Part model, mm, in its own coordinate system. A direction names the side the tool comes from. Coordinates: 2 decimals unless noted, no trailing zeros. Use a Markdown table: item, result. Add a question column.
1. Pull direction Y, two halves, no side cores. Call faces 3 (the flat face through (-5, 8, 0)), 4 (the flat face through (-6.4, 9.2, 0)), 5 (the cylindrical face through (-1.438, 10.955, -6.261)): pulls with the +Y half, pulls with the -Y half, needs draft (parallel to the pull), parting line crosses it, or undercut.
2. Drop flat-ended pins along their axis: pin 1 (10 mm diameter, centred on y = -9, z = 2, fed in from +X); pin 2 (6 mm diameter, centred on x = -5, z = 7, fed in from -Y); pin 3 (3 mm diameter, centred on y = -8, z = 37, fed in from +X). Give the stop position or say it passes through.
3. 3-axis set-ups, long thin cutter, end or side, ignore diameter. For faces 1 (the cylindrical face through (-1.88, -8.48, -6.26)), 2 (the flat face through (-7, -6, -12.7)): which of +Z, -Z, +X, -X, +Y, -Y reach the whole face in a straight line?
4. Wall check: probe 1 along Y at (x, z) = (0, -6.25); probe 2 along Y at (x, z) = (3.75, -2.5); probe 3 along X at (y, z) = (-8.5, 5). Give the ranges that are in metal, low to high. Write a range as [from, to].
from build123d import *

# Parameters (mm, degrees)
F2_R     = 11.049
F2_R_2   = 8.6868
F3_DEPTH = 12.7
F7_DEPTH = 3.302


# Not quite as in the source:
# - the program builds the solid bodies; features that only make, move or delete a surface that nothing else refers to are left out


with BuildPart() as f1:
    # F0 (on Front) → F1 (revolve)
    with BuildSketch(Plane.XZ):
        with BuildLine():
            Line((0, 59.2769769434), (0, 66.04))
            ThreePointArc((0, 66.04), (-9.3545638677, 33.6071762807), (-12.5095, 0))
            Line((-12.5095, 0), (-10.1473, 0))
            ThreePointArc((-10.1473, 0), (-7.5921575539, 30.0696179426), (0, 59.2769769434))
        make_face()
    revolve(axis=Axis((0, 0, 62.6584884717), (0, 0, 1)))

    # F2 (on Top) → F3 (join)
    with BuildSketch(Plane.XY):
        Circle(F2_R)
        Circle(F2_R_2, mode=Mode.SUBTRACT)
    extrude(amount=-F3_DEPTH)

    # F6 (on Front) → F7 (cut, symmetric)
    with BuildSketch(Plane.XZ):
        with BuildLine():
            ThreePointArc((6.9723, 0), (5.2204583943, 24.7022854782), (0, 48.9101079951))
            ThreePointArc((0, 48.9101079951), (-5.2204583943, 24.7022854782), (-6.9723, 0))
            Line((-6.9723, 0), (0, 0))
            Line((0, 0), (6.9723, 0))
        make_face()
    extrude(amount=F7_DEPTH, both=True, mode=Mode.SUBTRACT)


solid = f1.part
Geometry check:
| question | item | result |
|---|---|---|
| 1 | face 3 | undercut |
| 1 | face 4 | needs draft |
| 1 | face 5 | parting line crosses it |
| 2 | pin 1 | stops at x = 11.84 |
| 2 | pin 2 | stops at y = -12.22 |
| 2 | pin 3 | stops at x = 5.81 |
| 3 | face 1 | -Z |
| 3 | face 2 | -Z, +X, -X, +Y, -Y |
| 4 | probe 1 | y = [-11.05, -8.69], [8.69, 11.05] |
| 4 | probe 2 | y = [-10.39, -7.84], [7.84, 10.39] |
| 4 | probe 3 | x = [-9.08, -5.41], [5.41, 9.08] |
